from build123d import *

# Parameters (mm, degrees)
SKETCH001_R  = 7.071068
PAD001_DEPTH = 225
SKETCH002_R  = 15
PAD002_DEPTH = 75
PAD002_TAPER = 2.5
FILLET001_R  = 2
FILLET002_R  = 5


with BuildPart() as part:
    # Sketch001 → Pad001 (new body)
    with BuildSketch(Plane.XY):
        with Locations((15, 0)):
            Circle(SKETCH001_R)
    extrude(amount=PAD001_DEPTH)

    # Sketch002 → Pad002 (join)
    with BuildSketch(Plane.XY.offset(225)):
        with Locations((15, 0)):
            Circle(SKETCH002_R)
    extrude(amount=-PAD002_DEPTH, taper=PAD002_TAPER)

    # Fillet001
    fillet001_edges = [part.edges().sort_by_distance(p)[0] for p in [
        (7.928932, 0, 0),
        (7.928932, 0, 150),
        (3.274571, 0, 150),
    ]]
    fillet(fillet001_edges, radius=FILLET001_R)

    # Fillet002
    fillet002_edges = [part.edges().sort_by_distance(p)[0] for p in [
        (0, 0, 225),
    ]]
    fillet(fillet002_edges, radius=FILLET002_R)


solid = part.part
Model file for the job. Use its own axes, mm. A direction names the side the tool comes from. Give positions to 0.01 mm unless a question says otherwise; leave off trailing zeros. Order: outer loops, then holes, each group sorted by start corner. A loop starts at its lowest first (then second) coordinate and runs counter-clockwise, first axis right, second up. Notation, with made-up numbers: M -33.75,6 L -3.75,6 A26 cw -3.75,43 Z; hole C 72.25,36.25 d4. An arc over 180 degrees is marked long. Put each result on its own line as item: value. Start each with the question number.
(1) Pin check, flat tips, straight feed: pin 1 Ø3 at (y, z) = (-11, 171.5) entering from -X; pin 2 Ø4 at (x, z) = (22, 34.5) entering from +Y; pin 3 Ø8 at (x, y) = (20, 11) entering from -Z. Stop position of each tip, or through.
(2) Band-saw the part on A-A on x = 15. Give the cut face in (y, z).
(3) Band-saw the part on B-B on z = 65.5. Give the cut face in (x, y), then the cut area to 3 significant figures.
(4) Tool access for faces 1 (the face through (21.745, 2.124, 73.978)), 2 (the face through (15, 0, 0)): list every direction of +Z, -Z, +X, -X, +Y, -Y with a clear straight run to the whole face (end or side of a thin tool).
(5) Band-saw the part on C-C on z = 155.5. Give the cut face in (x, y).
(6) Drill centre lines: L1, parallel to X at y = -0.25, z = 96.5; L2, parallel to Y at x = 4.5, z = 168; L3, parallel to X at y = 5.5, z = 67. Where is each one in solid material? Low to high. Write a range as [from, to].
Results below:
1. pin 1: stops at x = 6.62
1. pin 2: stops at y = 5
1. pin 3: stops at z = 149.74
2. outline: M -14.77,219.78 L -11.81,151.91 A2 ccw -9.81,150 L -9.07,150 A2 cw -7.07,148 L -7.07,2 A2 ccw -5.07,0 L 5.07,0 A2 ccw 7.07,2 L 7.07,148 A2 cw 9.07,150 L 9.81,150 A2 ccw 11.81,151.91 L 14.77,219.78 A5 ccw 9.78,225 L -9.78,225 A5 ccw Z
3. outline: C 15,0 d14.14
3. area: 157 mm2
4. face 1: -Z
4. face 2: -Z, +X, -X, +Y, -Y
5. outline: C 15,0 d23.93
6. L1: x = [7.93, 22.07]
6. L2: y = [-6.8, 6.8]
6. L3: x = [10.56, 19.44]
